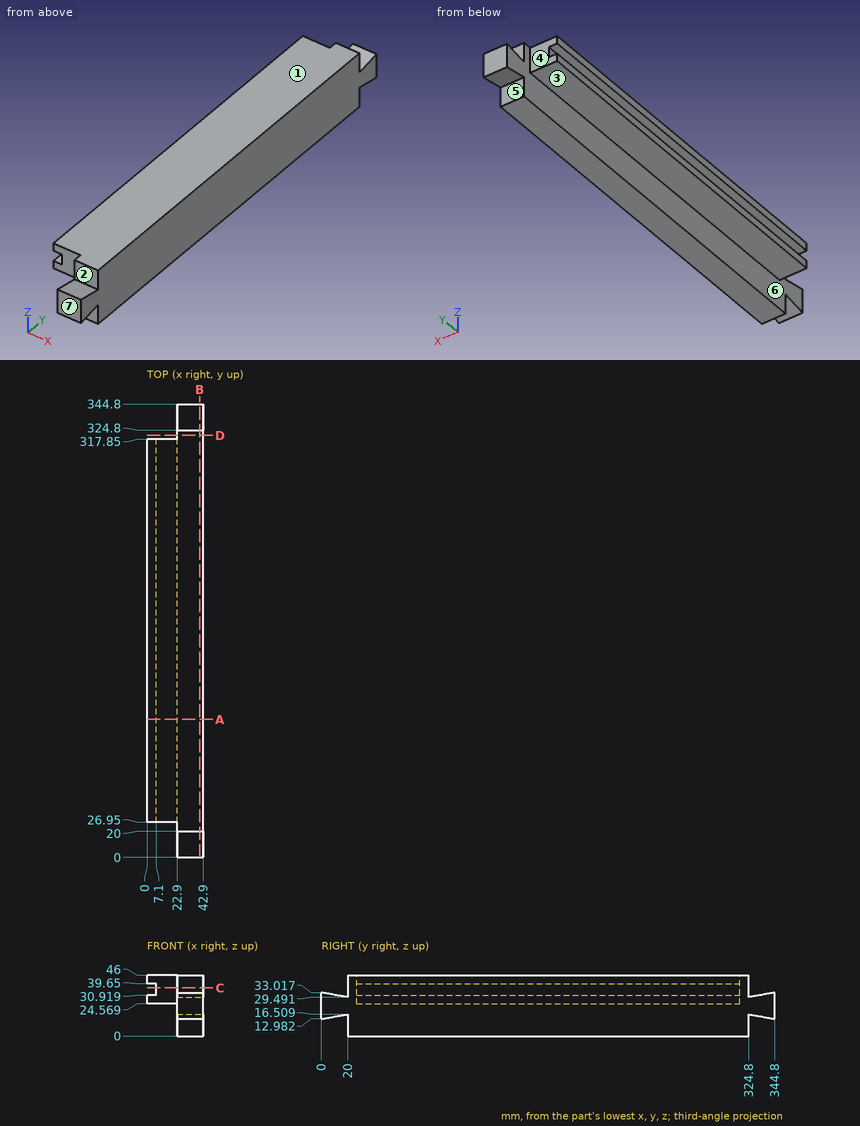
Geometry: see drawing. Coordinates: mm, zero at the bounding-box minimum. A direction names the side the tool comes from. Coordinates: 2 decimals unless noted, no trailing zeros. Loops run counter-clockwise (first coordinate to the right, second up) from the corner with the lowest first, then second, coordinate; pieces in that order, holes last. Notation, with made-up numbers: (-15, -7) -> (-10, -7) arc R29 ccw to (-10, 32) -> close; hole circle Ø8 at (11, 66.25). An arc over 180 degrees is marked (long way). Use a Markdown table: item, result.
1) Access query for the marked faces 1, 2, 3 and 4. Directions: +Z, -Z, +X, -X, +Y, -Y. A direction counts if a zero-diameter tool reaches every point of the face in a straight line with its end or side. Return the directions, or none.
Results found:
| item | result |
|---|---|
| face 1 | +Z, +X, -X, +Y, -Y |
| face 2 | +Z, +X, -X |
| face 3 | -Z, -X, +Y, -Y |
| face 4 | +Z, -Z, -X, +Y |
2) Pull-direction query (Y, two-part tool) for the marked faces 5, 6 and 7; classes: released by +Y, released by -Y, zero draft, split by the parting line, or undercut.
Results found:
| item | result |
|---|---|
| face 5 | undercut |
| face 6 | zero draft |
| face 7 | released by -Y |
3) Contact query for flat-ended pins moving along their axis: pin 1 (8.5 mm diameter, centred on x = 37.5, z = 5, fed in from -Y); pin 2 (1.5 mm diameter, centred on y = 185, z = 23.5, fed in from -X); pin 3 (23.5 mm diameter, centred on x = 8.5, z = 40, fed in from +Y). Output: stop coordinate, or through.
Results found:
| item | result |
|---|---|
| pin 1 | stops at y = 20 |
| pin 2 | stops at x = 22.9 |
| pin 3 | stops at y = 317.85 |
4) Cut plane D-D (y = 321). Return the cut outline in (x, z), then the cut area to 3 significant figures.
Results found:
| item | result |
|---|---|
| outline | (22.9, 0) -> (42.9, 0) -> (42.9, 46) -> (22.9, 46) -> close |
| area | 920 mm2 |
5) Cut plane A-A (y = 105). Return the cut outline in (x, z), then the cut area to 3 significant figures.
Results found:
| item | result |
|---|---|
| outline | (0, 24.57) -> (22.9, 24.57) -> (22.9, 0) -> (42.9, 0) -> (42.9, 46) -> (0, 46) -> (0, 39.65) -> (7.1, 39.65) -> (7.1, 30.92) -> (0, 30.92) -> close |
| area | 1,350 mm2 |
6) Cut plane C-C (z = 36.5). Return the cut outline in (x, y).
Results found:
| item | result |
|---|---|
| outline | (7.1, 26.95) -> (22.9, 26.95) -> (22.9, 20) -> (42.9, 20) -> (42.9, 324.8) -> (22.9, 324.8) -> (22.9, 317.85) -> (7.1, 317.85) -> close |
7) Cut plane B-B (x = 40). Return the cut outline in (y, z), then the cut area to 3 significant figures.
Results found:
| item | result |
|---|---|
| outline | (0, 12.98) -> (20, 16.51) -> (20, 0) -> (324.8, 0) -> (324.8, 16.51) -> (344.8, 12.98) -> (344.8, 33.02) -> (324.8, 29.49) -> (324.8, 46) -> (20, 46) -> (20, 29.49) -> (0, 33.02) -> close |
| area | 14,700 mm2 |
8) Material intervals for line 1 along Y through (x, z) = (4, 29); line 2 along X through (y, z) = (144, 17.5); line 3 along Z through (x, y) = (6, 132.5), sorted ascending. Write a range as from..to.
Results found:
| item | result |
|---|---|
| line 1 | y = 26.95..317.85 |
| line 2 | x = 22.9..42.9 |
| line 3 | z = 24.57..30.92, 39.65..46 |
